from build123d import *

# Parameters (mm, degrees)
SKETCH_1_W          = 170
SKETCH_1_H          = 40
EXTRUDE_1_DEPTH     = 2
SKETCH_2_R          = 2.5
CUT_EXTRUDE_1_DEPTH = 88.344146913
SKETCH_3_R          = 1.5
CUT_EXTRUDE_2_DEPTH = 88.344146913
FILLET_1_R          = 3


with BuildPart() as part:
    # 草图1 → 凸台-拉伸1 (new body)
    with BuildSketch(Plane(origin=(0, 0, 0), x_dir=(0, 0, -1), z_dir=(1, 0, 0))):
        Rectangle(SKETCH_1_W, SKETCH_1_H)
    extrude(amount=EXTRUDE_1_DEPTH)

    # 草图2 → 切除-拉伸1 (cut, through all)
    with BuildSketch(Plane(origin=(2, 0, 0), x_dir=(0, 0, -1), z_dir=(1, 0, 0))):
        with Locations((-75, 12.5)):
            Circle(SKETCH_2_R)
        with Locations(Location((-75, -12.5, 0), (0, 0, 180))):
            Circle(SKETCH_2_R)
        with Locations((75, -12.5)):
            Circle(SKETCH_2_R)
        with Locations(Location((75, 12.5, 0), (0, 0, 180))):
            Circle(SKETCH_2_R)
    extrude(amount=-CUT_EXTRUDE_1_DEPTH, mode=Mode.SUBTRACT)

    # 草图3 → 切除-拉伸2 (cut, through all)
    with BuildSketch(Plane(origin=(2, 0, 0), x_dir=(0, 0, -1), z_dir=(1, 0, 0))):
        with Locations((-37.5, 11)):
            Circle(SKETCH_3_R)
        with Locations((-37.5, -11)):
            Circle(SKETCH_3_R)
        with Locations((37.5, 11)):
            Circle(SKETCH_3_R)
        with Locations((37.5, -11)):
            Circle(SKETCH_3_R)
    extrude(amount=-CUT_EXTRUDE_2_DEPTH, mode=Mode.SUBTRACT)

    # 圆角1
    fillet_1_edges = [part.edges().sort_by_distance(p)[0] for p in [
        (1, -20, -85),
        (1, -20, 85),
        (1, 20, 85),
        (1, 20, -85),
    ]]
    fillet(fillet_1_edges, radius=FILLET_1_R)


solid = part.part
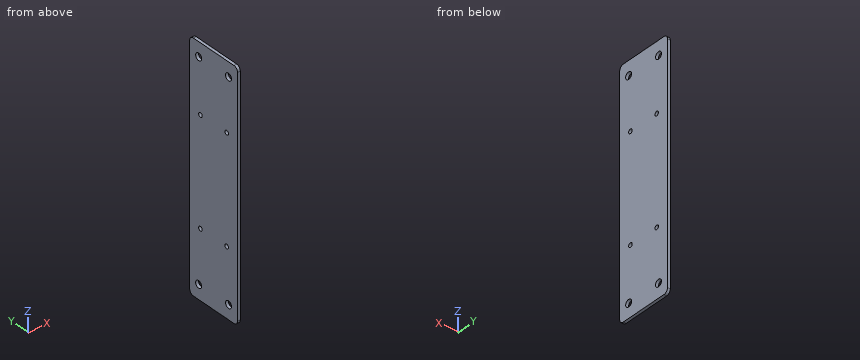
Check sheet for the modelled part. Datum: model origin and axes. Units: mm. Coordinates: 2 decimals unless noted, no trailing zeros. Loops run counter-clockwise (first coordinate to the right, second up) from the corner with the lowest first, then second, coordinate; pieces in that order, holes last. Notation, with made-up numbers: (-9.75, 26.5) -> (6.25, 26.5) arc R28 cw to (6.25, 59.5) -> close; hole circle Ø8 at (-37, 22.5). An arc over 180 degrees is marked (long way). Answer in a Markdown table with one row per item.
1. Go/stop test with a flat-tipped pin: pin 1 (1.8 mm diameter, centred on y = -11, z = 37.5, fed in from -X). Record where the tip stops, or that it passes through.
Check values:
| item | result |
|---|---|
| pin 1 | passes through |
2. Sectioned sample at A-A, the plane z = 37.5. Record the boundary of the cut face in (x, y).
Check values:
| item | result |
|---|---|
| outline | (0, -20) -> (2, -20) -> (2, -12.5) -> (0, -12.5) -> close; (0, -9.5) -> (2, -9.5) -> (2, 9.5) -> (0, 9.5) -> close; (0, 12.5) -> (2, 12.5) -> (2, 20) -> (0, 20) -> close |
3. Material ranges on line 1 along Y through (x, z) = (0.7, -37.5); line 2 along Y through (x, z) = (0.8, -75); line 3 along Z through (x, y) = (1.7, 18.5), recorded low to high. Write a range as [from, to].
Check values:
| item | result |
|---|---|
| line 1 | y = [-20, -12.5], [-9.5, 9.5], [12.5, 20] |
| line 2 | y = [-20, -15], [-10, 10], [15, 20] |
| line 3 | z = [-84.6, 84.6] |
4. Sectioned sample at C-C, the plane z = 75. Record the boundary of the cut face in (x, y), then the cut area to 3 significant figures.
Check values:
| item | result |
|---|---|
| outline | (0, -20) -> (2, -20) -> (2, -15) -> (0, -15) -> close; (0, -10) -> (2, -10) -> (2, 10) -> (0, 10) -> close; (0, 15) -> (2, 15) -> (2, 20) -> (0, 20) -> close |
| area | 60.0 mm2 |
5. Sectioned sample at B-B, the plane x = 1.4. Give the number of separate pieces and of enclosed holes in the cut face, then the cut area to 3 significant figures.
Check values:
| item | result |
|---|---|
| separate pieces | 1 |
| enclosed holes | 8 |
| area | 6,690 mm2 |
